The listing builds one solid part. Answer for the finished solid, in the listing's coordinates (mm). A direction names the side the tool comes from. Coordinates: 2 decimals unless noted, no trailing zeros. Order: outer loops, then holes, each group sorted by start corner. A loop starts at its lowest first (then second) coordinate and runs counter-clockwise, first axis right, second up. Notation, with made-up numbers: (64.25, 23) -> (103.25, 23) arc R30 cw to (103.25, 51) -> close; hole circle Ø1 at (18, -29). An arc over 180 degrees is marked (long way). Write each question's results on one line, items separated by ' | '. Start each with the question number.
(1) Given pin 1 (0.9 mm diameter, centred on x = 24.5, z = 12, fed in from -Y); pin 2 (12 mm diameter, centred on x = 21, y = 44, fed in from -Z); pin 3 (6.5 mm diameter, centred on x = 15, z = 12, fed in from +Y); pin 4 (5 mm diameter, centred on x = 13, y = 27.5, fed in from +Z), each flat-ended and moving along its own axis, determine where each tip first touches the part or whether it passes through.
(2) The part is cut by section B-B, the plane x = 20. Give the vertices of the cut face in (y, z).
(3) The part is cut by section C-C, the plane x = 23. Give the vertices of the cut face in (y, z), then the cut area to 3 significant figures.
(4) Straight lines are drawn through the part: L1, parallel to Y at x = 20.5, z = 2.75; L2, parallel to X at y = -1.5, z = 10.5; L3, parallel to Z at x = 26, y = 57.5. For each, find the intervals that lie inside material, in ascending order.
(5) The part is cut by section D-D, the plane z = 6. Give the vertices of the cut face in (x, y), then the cut area to 3 significant figures.
(6) Determine the mould class of faces 1 (the face through (15, 65, 3)), 2 (the face through (15, -5, 8)), 3 (the face through (12.54, 43.45, 3.55)) for opening direction Y: +Y half, -Y half, draft (parallel to the pull), parting line (faces both ways), or undercut.
(7) The part is cut by section A-A, the plane y = 59. Give the vertices of the cut face in (x, z), then the cut area to 3 significant figures.
(8) A tool of negligible diameter and unlimited length cuts with its end or side. For faces 4 (the face through (25.003, -2.535, 12.631)), 5 (the face through (30, 20, 5)), 6 (the face through (15, 33, 7)), from which of +Z, -Z, +X, -X, +Y, -Y can it reach the whole face along a straight path? Write none if from no direction.
```python
from build123d import *

# Parameters (mm, degrees)
SKETCH_W        = 30
SKETCH_H        = 65
PAD_DEPTH       = 7
SKETCH001_W     = 5
SKETCH001_H     = 17
PAD001_DEPTH    = 30
PAD002_DEPTH    = 6
PAD003_DEPTH    = 6
SKETCH004_R     = 2.1
POCKET_DEPTH    = 12
SKETCH005_R     = 2.1
POCKET001_DEPTH = 5
FILLET_R        = 5


with BuildPart() as part:
    # Sketch → Pad (new body)
    with BuildSketch(Plane.XY):
        with Locations((15, 32.5)):
            Rectangle(SKETCH_W, SKETCH_H)
    extrude(amount=PAD_DEPTH)

    # Sketch001 (on DatumPlane) → Pad001 (join)
    with BuildSketch(Plane.YZ.offset(30)):
        with Locations((-2.5, 8.5)):
            Rectangle(SKETCH001_W, SKETCH001_H)
    extrude(amount=-PAD001_DEPTH)

    # Sketch002 (on DatumPlane) → Pad002 (join)
    with BuildSketch(Plane.YZ.offset(30)):
        Polygon((0, 17), (0, 7), (15, 7), align=None)
    extrude(amount=-PAD002_DEPTH)

    # Sketch003 (on DatumPlane) → Pad003 (join)
    with BuildSketch(Plane(origin=(0, 0, 0), x_dir=(0, -1, 0), z_dir=(-1, 0, 0))):
        Polygon((0, 17), (0, 7), (-15, 7), align=None)
    extrude(amount=-PAD003_DEPTH)

    # Sketch004 (on Face6 of Pad003) → Pocket (cut)
    with BuildSketch(Plane.XY.offset(7)):
        with Locations((20, 59)):
            Circle(SKETCH004_R)
        with Locations((20, 32)):
            Circle(SKETCH004_R)
        with Locations((13, 45.5)):
            Circle(SKETCH004_R)
    extrude(amount=-POCKET_DEPTH, mode=Mode.SUBTRACT)

    # Sketch005 (on Face8 of Pocket) → Pocket001 (cut)
    with BuildSketch(Plane.XZ.offset(5)):
        with Locations((7.000014, 11.981068)):
            Circle(SKETCH005_R)
        with Locations((15.000001, 11.995259)):
            Circle(SKETCH005_R)
        with Locations((23, 12)):
            Circle(SKETCH005_R)
    extrude(amount=-POCKET001_DEPTH, mode=Mode.SUBTRACT)

    # Fillet
    fillet_edges = [part.edges().sort_by_distance(p)[0] for p in [
        (0, 65, 3.5),
        (30, 65, 3.5),
    ]]
    fillet(fillet_edges, radius=FILLET_R)


solid = part.part
```
Established:
1) pin 1: stops at y = 0 | pin 2: stops at z = 0 | pin 3: stops at y = 0 | pin 4: stops at z = 7
2) outline: (-5, 0) -> (29.9, 0) -> (29.9, 7) -> (0, 7) -> (0, 17) -> (-5, 17) -> close; (34.1, 0) -> (56.9, 0) -> (56.9, 7) -> (34.1, 7) -> close; (61.1, 0) -> (65, 0) -> (65, 7) -> (61.1, 7) -> close
3) outline: (-5, 0) -> (65, 0) -> (65, 7) -> (0, 7) -> (0, 9.9) -> (-5, 9.9) -> close; (-5, 14.1) -> (0, 14.1) -> (0, 17) -> (-5, 17) -> close | area: 519 mm^2
4) L1: y = -5 to 29.96, 34.04 to 56.96, 61.04 to 65 | L2: x = 0 to 5.51, 8.49 to 13.53, 16.47 to 21.53, 24.47 to 30 | L3: z = 0 to 7
5) outline: (0, -5) -> (30, -5) -> (30, 60) arc R5 ccw to (25, 65) -> (5, 65) arc R5 ccw to (0, 60) -> close; hole circle Ø4.2 at (13, 45.5); hole circle Ø4.2 at (20, 32); hole circle Ø4.2 at (20, 59) | area: 2,050 mm^2
6) face 1: +Y half | face 2: -Y half | face 3: undercut
7) outline: (0, 0) -> (17.9, 0) -> (17.9, 7) -> (0, 7) -> close; (22.1, 0) -> (30, 0) -> (30, 7) -> (22.1, 7) -> close | area: 181 mm^2
8) face 4: -Y | face 5: +Z, -Z, +X, +Y, -Y | face 6: +Z, +Y
